Geometry: final body of the model. Coordinates: model frame, mm. Face numbers are marked on the shaded views. A direction names the side the tool comes from. Give positions to 0.01 mm unless a question says otherwise; leave off trailing zeros. Order: outer loops, then holes, each group sorted by start corner. A loop starts at its lowest first (then second) coordinate and runs counter-clockwise, first axis right, second up. Notation, with made-up numbers: (26, 9.25) - (67, 9.25) arc R25 cw to (67, 42.25) - close; hole circle Ø8 at (-2, -21.5). An arc over 180 degrees is marked (long way). One line per question, with ' | ' between items. Start each with the question number.
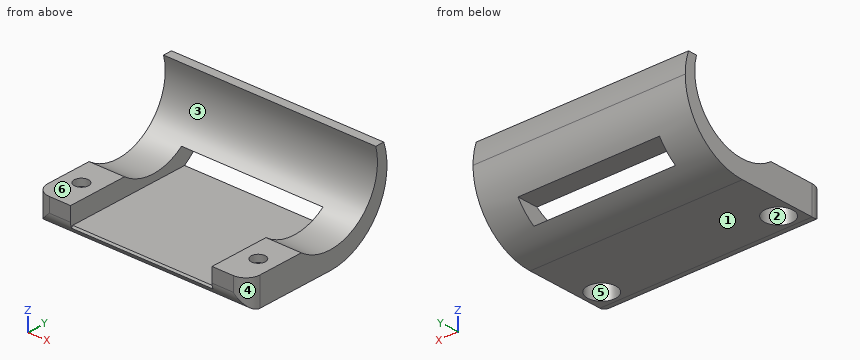
from build123d import *

# Parameters (mm, degrees)
F0_W            = 30
F0_H            = 22
F1_DEPTH        = 12
F3_DEPTH        = 30.001
F3_DEPTH_BACK   = 25
F5_START        = -25
F5_DEPTH        = 40.001
F6_R            = 2
F7_W            = 20
F7_H            = 34.384613307
F8_DEPTH        = 2.5
F9_T1_DEPTH     = 20
F11_D           = 2
F11_DEPTH       = 8
F11_CBORE_D     = 4
F11_CBORE_DEPTH = 3
F11_TIP         = 0.600860619


# Not quite as in the source:
# - a fillet or chamfer that OpenCascade refuses, or shapes differently, is made with other operations: its cross-section is extruded or revolved along the edge and cut away or added


with BuildPart() as f1:
    # F0 (on Top) → F1 (new body)
    with BuildSketch(Plane.XY):
        Rectangle(F0_W, F0_H)
    extrude(amount=F1_DEPTH)

    # F2 (on face) → F3 (cut, two sides)
    with BuildSketch(Plane(origin=(-15, 0, 0), x_dir=(0, -1, 0), z_dir=(-1, 0, 0))) as f3_sk:
        with BuildLine():
            ThreePointArc((2.5, 4), (4.7082039325, 6.6458980338), (5.5, 10))
            ThreePointArc((5.5, 10), (3.3033008589, 15.3033008589), (-2, 17.5))
            Line((-2, 17.5), (-2, 4))
            Line((-2, 4), (2.5, 4))
        make_face()
        with BuildLine():
            ThreePointArc((-2, 17.5), (3.3033008589, 15.3033008589), (5.5, 10))
            ThreePointArc((5.5, 10), (4.7082039325, 6.6458980338), (2.5, 4))
            Line((2.5, 4), (15.6530104578, 4))
            Line((15.6530104578, 4), (15.6530104578, 18.6757147312))
            Line((15.6530104578, 18.6757147312), (-2, 18.6757147312))
            Line((-2, 18.6757147312), (-2, 17.5))
        make_face()
        with BuildLine():
            Line((-2, 4), (-2, 17.5))
            ThreePointArc((-2, 17.5), (-9.1151247354, 7.6282917549), (2.5, 4))
            Line((2.5, 4), (-2, 4))
        make_face()
    extrude(amount=-F3_DEPTH, mode=Mode.SUBTRACT)
    extrude(f3_sk.sketch, amount=F3_DEPTH_BACK, mode=Mode.SUBTRACT)

    # F4 (on Right) → F5 (intersect)
    with BuildSketch(Plane.YZ.offset(F5_START)):
        with BuildLine():
            ThreePointArc((2, 0), (8.3639610307, 2.6360389693), (11, 9))
            ThreePointArc((11, 9), (8.3639610307, 15.3639610307), (2, 18))
            Line((2, 18), (2, 0))
        make_face()
        with BuildLine():
            Line((2, 0), (2, 18))
            ThreePointArc((2, 18), (-7, 9), (2, 0))
        make_face()
        with BuildLine():
            ThreePointArc((2, 0), (-7, 9), (2, 18))
            Line((2, 18), (2, 22.4318560213))
            Line((2, 22.4318560213), (-24.2340825498, 22.4318560213))
            Line((-24.2340825498, 22.4318560213), (-24.2340825498, -9.0490430593))
            Line((-24.2340825498, -9.0490430593), (2, -9.0490430593))
            Line((2, -9.0490430593), (2, 0))
        make_face()
    extrude(amount=F5_DEPTH, mode=Mode.INTERSECT)

    # F6
    f6_edges = [f1.edges().sort_by_distance(p)[0] for p in [
        (0, -11, 0),
        (-15, -11, 2),
        (15, -11, 2),
    ]]
    fillet(f6_edges, radius=F6_R)

    # F7 (on face) → F8 (cut)
    with BuildSketch(Plane.XY.offset(4)):
        with Locations((0, -1.0834368877)):
            Rectangle(F7_W, F7_H)
    extrude(amount=-F8_DEPTH, mode=Mode.SUBTRACT)

    # F9: chamfer of 0.25 on 1 edges, made by hand

    # F9_s2 → F9_t1 (cut)
    with BuildSketch(Plane.YZ.offset(-10)):
        with BuildLine():
            Line((-10.8522111232, 1.2236697613), (-10.662309407, 1.5083186711))
            Line((-10.662309407, 1.5083186711), (-10.662309407, 1.5133186711))
            ThreePointArc((-10.662309407, 1.5133186711), (-10.7994005401, 1.505), (-10.9364916731, 1.505))
            Line((-10.9364916731, 1.505), (-10.9413329023, 1.49875))
            ThreePointArc((-10.9413329023, 1.49875), (-10.9000798671, 1.3599050861), (-10.8568277766, 1.2217497324))
            Line((-10.8568277766, 1.2217497324), (-10.8522111232, 1.2236697613))
        make_face()
    extrude(amount=F9_T1_DEPTH, mode=Mode.SUBTRACT)

    # F11
    with Locations(Plane(origin=(0, 0, 0), x_dir=(1, 0, 0), z_dir=(0, 0, -1))):
        with Locations((12.5, 6.5), (-12.5, 6.5)):
            CounterBoreHole(F11_D / 2, F11_CBORE_D / 2, F11_CBORE_DEPTH, depth=F11_DEPTH)
            with Locations((0, 0, -(F11_DEPTH + F11_TIP / 2))):  # 118° drill point
                Cone(0, F11_D / 2, F11_TIP, mode=Mode.SUBTRACT)


solid = f1.part
(1) Cut plane B-B, the plane y = -6.5. Return the cut outline in (x, z).
(2) Cut plane C-C, the plane x = -12.5. Return the cut outline in (y, z).
(3) Contact query for flat-ended pins moving along their axis: P1, Ø3.5, axis at x = -12.5, y = -6.5, coming from the -Z side; P2, Ø9, axis at x = -3.5, y = 1.5, coming from the +Z side; P3, Ø4, axis at y = -0.5, z = 6, coming from the +X side; P4, Ø4, axis at x = -12, y = -7.5, coming from the +Z side. Output: stop coordinate, or through.
(4) Pull-direction query (Z, two-part tool) for the marked faces 1, 2 and 3; classes: +Z half, -Z half, draft (parallel to the pull), parting line (faces both ways), or undercut.
(5) Material intervals for line 1 along X through (y, z) = (-6.5, 3.8); line 2 along X through (y, z) = (-8.25, 1.25); line 3 along Y through (x, z) = (12.5, 3.2), sorted ascending. Write a range as from..to.
(6) Access query for the marked faces 4, 5 and 6. Directions: +Z, -Z, +X, -X, +Y, -Y. A direction counts if a zero-diameter tool reaches every point of the face in a straight line with its end or side. Return the directions, or none.
(7) Cut plane A-A, the plane x = 1.25. Return the cut outline in (y, z).
(8) Cut plane D-D, the plane y = 7.75. Return the cut outline in (x, z).
Results are:
1) outline: (-15, 0) - (-14.5, 0) - (-14.5, 3) - (-13.5, 3) - (-13.5, 4) - (-15, 4) - close; (-11.5, 3) - (-10.5, 3) - (-10.5, 0) - (10.5, 0) - (10.5, 3) - (11.5, 3) - (11.5, 4) - (10, 4) - (10, 1.5) - (-10, 1.5) - (-10, 4) - (-11.5, 4) - close; (13.5, 3) - (14.5, 3) - (14.5, 0) - (15, 0) - (15, 4) - (13.5, 4) - close
2) outline: (-11, 2) arc R2 ccw to (-9, 0) - (-8.5, 0) - (-8.5, 3) - (-7.5, 3) - (-7.5, 4) - (-11, 4) - close; (-5.5, 3) - (-4.5, 3) - (-4.5, 0) - (2, 0) arc R9 ccw to (10.49, 12) - (9.23, 12) arc R7.5 cw to (-2.5, 4) - (-5.5, 4) - close
3) P1: z = 3 | P2: z = 1.5 | P3: through | P4: z = 4
4) face 1: -Z half | face 2: draft | face 3: undercut
5) line 1: -15..-13.5, -11.5..-10, 10..11.5, 13.5..15 | line 2: -15..-13.47, -11.53..11.53, 13.47..15 | line 3: -11..-7.5, -5.5..-1.16, 5.16..8.88
6) face 4: +Z, -Z, +X, -Y | face 5: -Z | face 6: +Z, +X, -X, -Y
7) outline: (-10.85, 1.23) arc R2 ccw to (-9, 0) - (2, 0) arc R9 ccw to (6.97, 1.5) - (-10.67, 1.5) - close; (6.5, 4) - (9.48, 4) arc R9 ccw to (10.49, 12) - (9.23, 12) arc R7.5 cw to start
8) outline: (-15, 2.08) - (-10, 2.08) - (-10, 4) - (10, 4) - (10, 2.08) - (15, 2.08) - (15, 5.18) - (-15, 5.18) - close
